Part model, mm, in its own coordinate system. Round coordinates to 2 decimals unless told otherwise and drop trailing zeros. Loops run counter-clockwise (first coordinate to the right, second up) from the corner with the lowest first, then second, coordinate; pieces in that order, holes last.
(1) Cut at A-A on x = 13. List the corners of the cut face in (y, z).
(2) Cut at B-B on y = 126. List the corners of the cut face in (x, z), then the cut area to 3 significant figures.
(3) Flat gauge pins, fed straight in: pin 1 (5 mm diameter, centred on x = -11, z = 12, fed in from +Y); pin 2 (1.5 mm diameter, centred on y = 154, z = -2, fed in from -X); pin 3 (6 mm diameter, centred on x = -7, y = -122.5, fed in from +Z). Where does each tip first touch, or does it go through?
(4) Cut at C-C on z = -13.5. List the corners of the cut face in (x, y).
(5) Probe probe 1 along Y at (x, z) = (-8, -15); probe 2 along X at (y, z) = (25, 2); probe 3 along X at (y, z) = (159, -21). List the from-to ranges inside material, lowest first.
from build123d import *

# Parameters (mm, degrees)
SKETCH1_R           = 24.0411
BOSS_EXTRUDE1_DEPTH = 211.0105
SKETCH2_R           = 9.017
BOSS_EXTRUDE2_DEPTH = 2.54
BOSS_EXTRUDE3_DEPTH = 18.415


with BuildPart() as part:
    # Sketch1 → Boss-Extrude1 (new body)
    with BuildSketch(Plane(origin=(0, 0, 0), x_dir=(1, 0, 0), z_dir=(0, 1, 0))):
        with Locations(Location((0, 0, 0), (0, 0, 270))):
            Circle(SKETCH1_R)
    boss_extrude1 = extrude(amount=BOSS_EXTRUDE1_DEPTH)

    # Sketch2 → Boss-Extrude2 (add)
    with BuildSketch(Plane(origin=(0, 211.0105, 0), x_dir=(1, 0, 0), z_dir=(0, 1, 0))):
        with Locations(Location((0, 0, 0), (0, 0, 270))):
            Circle(SKETCH2_R)
    boss_extrude2 = extrude(amount=BOSS_EXTRUDE2_DEPTH)

    # Sketch3 → Boss-Extrude3 (add)
    with BuildSketch(Plane(origin=(0, 213.5505, 0), x_dir=(1, 0, 0), z_dir=(0, 1, 0))):
        Polygon((5.963677607, -2.264512398), (4.942964068, 4.032440108), (-1.020713539, 6.296952507), (-5.963677607, 2.264512398), (-4.942964068, -4.032440108), (1.020713539, -6.296952507), align=None)
    boss_extrude3 = extrude(amount=BOSS_EXTRUDE3_DEPTH)

    # Mirror1: Boss-Extrude1, Boss-Extrude2, Boss-Extrude3 across plane
    add(boss_extrude1.mirror(Plane.ZX))
    add(boss_extrude2.mirror(Plane.ZX))
    add(boss_extrude3.mirror(Plane.ZX))


solid = part.part
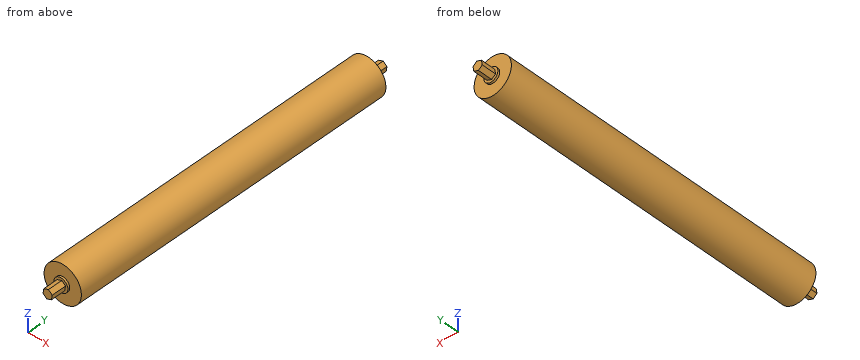
Final values:
1. outline: (-211.01, -20.22) - (211.01, -20.22) - (211.01, 20.22) - (-211.01, 20.22) - close
2. outline: circle Ø48.08 at (0, 0)
2. area: 1,820 mm2
3. pin 1: stops at y = 211.01
3. pin 2: stops at x = -24.01
3. pin 3: stops at z = 23.71
4. outline: (-19.89, -211.01) - (19.89, -211.01) - (19.89, 211.01) - (-19.89, 211.01) - close
5. probe 1: y = -211.01 to 211.01
5. probe 2: x = -23.96 to 23.96
5. probe 3: x = -11.7 to 11.7
